Job drawing, mm, ordinate dimensions from the low corner. One solid piece. Round coordinates to 2 decimals unless told otherwise and drop trailing zeros. Loops run counter-clockwise (first coordinate to the right, second up) from the corner with the lowest first, then second, coordinate; pieces in that order, holes last. Notation, with made-up numbers: M 20,63.5 L 76,63.5 A7 cw 76,69.5 Z; hole C 33,25.5 d4. An arc over 180 degrees is marked long. One line per item, written item: value.
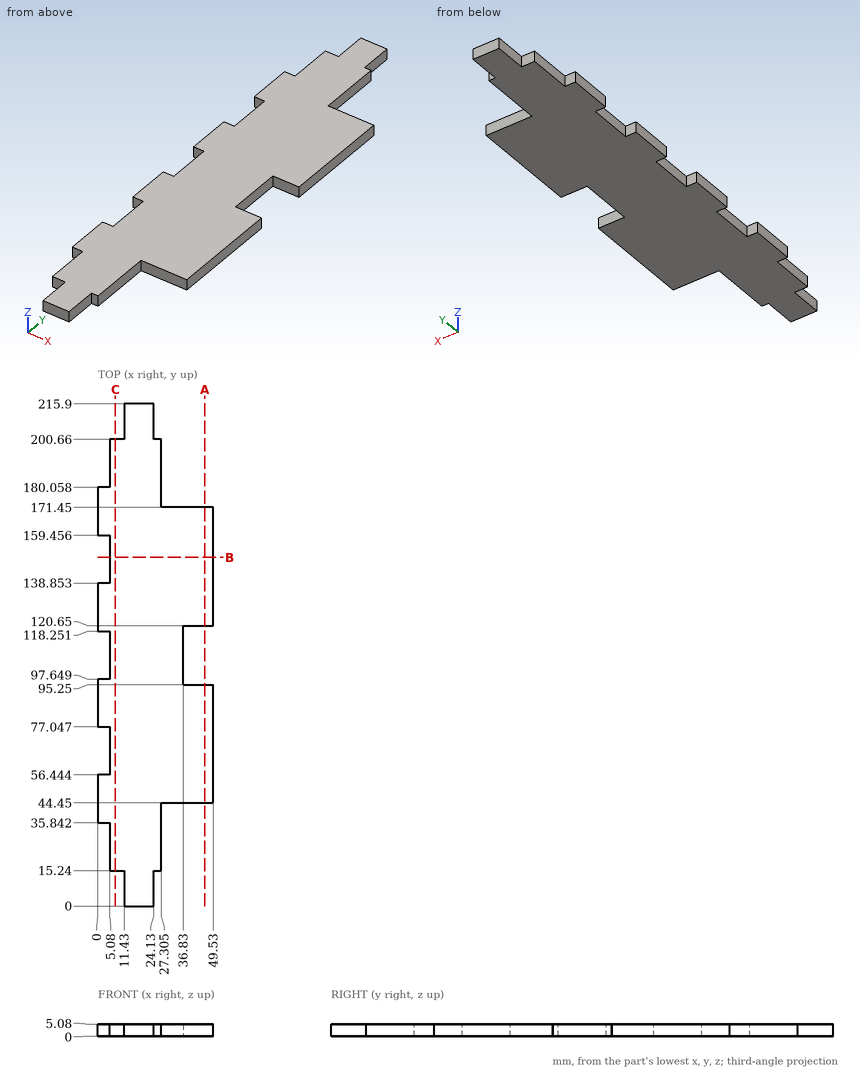
Item 1: Slice it at A-A, the plane x = 46. Give the cut face in (y, z).
Check values:
outline: M 44.45,0 L 95.25,0 L 95.25,5.08 L 44.45,5.08 Z; M 120.65,0 L 171.45,0 L 171.45,5.08 L 120.65,5.08 Z
Item 2: Slice it at B-B, the plane y = 150. Give the cut face in (x, z).
Check values:
outline: M 5.08,0 L 49.53,0 L 49.53,5.08 L 5.08,5.08 Z
Item 3: Drop flat-ended pins along their axis: P1, Ø3, axis at x = 28.5, z = 3.5, coming from the -Y side; P2, Ø1.5, axis at y = 32.5, z = 1.5, coming from the +X side (3 decimals); P3, Ø2, axis at y = 24, z = 1.5, coming from the -X side. Give the stop position or say it passes through.
Check values:
P1: stops at y = 15.24
P2: stops at x = 27.305
P3: stops at x = 5.08
Item 4: Slice it at C-C, the plane x = 7.5. Give the cut face in (y, z).
Check values:
outline: M 15.24,0 L 200.66,0 L 200.66,5.08 L 15.24,5.08 Z
Item 5: Wall check: line 1 along Y through (x, z) = (4.5, 2.55) (1 decimal); line 2 along Y through (x, z) = (41.5, 4.1); line 3 along X through (y, z) = (74, 2.8). Give the ranges that are in metal, low to high.
Check values:
line 1: y = 35.8 to 56.4, 77 to 97.6, 118.3 to 138.9, 159.5 to 180.1
line 2: y = 44.45 to 95.25, 120.65 to 171.45
line 3: x = 5.08 to 49.53
